Here's how the part is built. I have some questions about the finished solid (model axes, mm). A direction names the side the tool comes from. Round coordinates to 2 decimals unless told otherwise and drop trailing zeros. Order: outer loops, then holes, each group sorted by start corner. A loop starts at its lowest first (then second) coordinate and runs counter-clockwise, first axis right, second up. Notation, with made-up numbers: (66, -5) -> (114, -5) arc R28 ccw to (114, 22) -> close; hole circle Ø6 at (-25.5, 52). An arc over 180 degrees is marked (long way). Use a Markdown table: item, result. Add a question column.
(1) If I drill on probe 1 along Z at (x, y) = (-115, -34.5); probe 2 along Z at (x, y) = (21.5, -4); probe 3 along X at (y, z) = (-11, 61.5), over which ranges is the centre line in solid material (lowest first)?
(2) I want a section at A-A, the plane y = 0. Please give me the cut outline in (x, z).
(3) I want a section at C-C, the plane z = 149. Please give me the cut outline in (x, y).
(4) I want a section at D-D, the plane y = 149. Please give me the cut outline in (x, z), then the cut area to 3 significant figures.
(5) I want a section at B-B, the plane x = 0. Please give me the cut outline in (y, z), then the cut area to 3 significant figures.
(6) Thinking about a two-plate mould opening in Z: for faces 5 (the face through (-2, -51.937, -6)), 6 (the face through (-2.75, -12.4, 90.79)), 7 (the face through (-2, 74, -12.7)), 8 (the face through (-1, 13, 196.85)), which applies, pulls with the +Z half, pulls with the -Z half, needs draft (parallel to the pull), parting line crosses it, or undercut?
(7) On a 3-axis mill with a long thin cutter (end or side, diameter ignored), from which of +Z, -Z, +X, -X, +Y, -Y can I reach the whole of each face in a straight line? I mean faces 1 (the face through (38.1, 0, 191)), 2 (the face through (-38.1, 0, 191)), 3 (the face through (-1, 19.05, 191)), 4 (the face through (-2.75, -12.4, 231.29)). Say none if no direction works.
(8) I'm going to push flat-ended pins straight in: P1, Ø5, axis at x = -29, z = 189.5, coming from the -Y side; P2, Ø5, axis at y = 9, z = 128, coming from the -X side; P3, Ø4, axis at y = 5, z = 191.5, coming from the +X side. Where does each tip first touch, or does it pass through?
from build123d import *

# Parameters (mm, degrees)
F0_R     = 12.7
F1_DEPTH = 266.7
F3_W     = 76.2
F3_H     = 38.1
F4_DEPTH = 12.7
F5_W     = 254
F5_H     = 255.137313
F6_DEPTH = 12.7


with BuildPart() as f1:
    # F0 (on Top) → F1 (new body)
    with BuildSketch(Plane.XY):
        Circle(F0_R)
    extrude(amount=F1_DEPTH)

    # F3 (on offset) → F4 (join)
    with BuildSketch(Plane.XY.offset(196.85)):
        Rectangle(F3_W, F3_H)
    extrude(amount=-F4_DEPTH)

    # F5 (on face) → F6 (join)
    with BuildSketch(Plane(origin=(0, 0, 0), x_dir=(1, 0, 0), z_dir=(0, 0, -1))):
        with Locations((0, -75.631343)):
            Rectangle(F5_W, F5_H)
    extrude(amount=F6_DEPTH)


solid = f1.part
Taken from the geometry:
| question | item | result |
|---|---|---|
| 1 | probe 1 | z = -12.7 to 0 |
| 1 | probe 2 | z = -12.7 to 0, 184.15 to 196.85 |
| 1 | probe 3 | x = -6.35 to 6.35 |
| 2 | outline | (-127, -12.7) -> (127, -12.7) -> (127, 0) -> (12.7, 0) -> (12.7, 184.15) -> (38.1, 184.15) -> (38.1, 196.85) -> (12.7, 196.85) -> (12.7, 266.7) -> (-12.7, 266.7) -> (-12.7, 196.85) -> (-38.1, 196.85) -> (-38.1, 184.15) -> (-12.7, 184.15) -> (-12.7, 0) -> (-127, 0) -> close |
| 3 | outline | circle Ø25.4 at (0, 0) |
| 4 | outline | (-127, -12.7) -> (127, -12.7) -> (127, 0) -> (-127, 0) -> close |
| 4 | area | 3,230 mm2 |
| 5 | outline | (-51.94, -12.7) -> (203.2, -12.7) -> (203.2, 0) -> (12.7, 0) -> (12.7, 184.15) -> (19.05, 184.15) -> (19.05, 196.85) -> (12.7, 196.85) -> (12.7, 266.7) -> (-12.7, 266.7) -> (-12.7, 196.85) -> (-19.05, 196.85) -> (-19.05, 184.15) -> (-12.7, 184.15) -> (-12.7, 0) -> (-51.94, 0) -> close |
| 5 | area | 10,200 mm2 |
| 6 | face 5 | needs draft |
| 6 | face 6 | undercut |
| 6 | face 7 | pulls with the -Z half |
| 6 | face 8 | pulls with the +Z half |
| 7 | face 1 | +Z, +X, +Y, -Y |
| 7 | face 2 | +Z, -X, +Y, -Y |
| 7 | face 3 | +Z, +X, -X, +Y |
| 7 | face 4 | +Z |
| 8 | P1 | stops at y = -19.05 |
| 8 | P2 | stops at x = -10.91 |
| 8 | P3 | stops at x = 38.1 |
